Autodesk Inventor part; units mm, degrees
ref_plane "YZ Plane" through (0, 0, 0) normal (1, 0, 0) x (0, 1, 0)
ref_plane "XZ Plane" through (0, 0, 0) normal (0, 1, 0) x (-1, 0, 0)
ref_plane "XY Plane" through (0, 0, 0) normal (0, 0, 1) x (1, 0, 0)
sketch "Sketch44" plane through (0, 0, 0) normal (0, 1, 0) x (-1, 0, 0)
  line L0 (-39.5, 120) -> (39.5, 120)
  line L1 (39.5, 120) -> (39.5, -120)
  line L2 (39.5, -120) -> (-39.5, -120)
  line L3 (-39.5, -120) -> (-39.5, 120)
  line L4 (-39.5, 120) -> (39.5, -120) construction
  line L5 (39.5, 120) -> (-39.5, -120) construction
  point P0 (0, 0)
  dimension "d138" = 79
  dimension "d139" = 240
extrude "Extrusion33" add sketch "Sketch44" along normal blind 3
sketch "Sketch45" plane through (0, 3, 0) normal (0, 1, 0) x (1, 0, 0)
  line L0 (35, -20) -> (-3, -20)
  line L1 (-3, -20) -> (-3, 20)
  line L2 (-3, 20) -> (35, 20)
  line L3 (35, 20) -> (35, -20)
  point P0 (0, 0)
  dimension "d142" = 38
  dimension "d143" = 40
extrude "Extrusion34" add sketch "Sketch45" along normal blind 30
sketch "Sketch46" plane through (0, 33, 0) normal (0, 1, 0) x (1, 0, 0)
  point P0 (0, 0)
sketch "Sketch47" plane through (0, 0, 0) normal (0, -1, 0) x (1, 0, 0)
  circle A0 centre (16, 0) radius 18
  point P0 (0, 0)
  dimension "d146" = 36
extrude "Extrusion35" cut sketch "Sketch47" against normal blind 30 draft -15
sketch "Sketch48" plane through (0, 33, 0) normal (0, 1, 0) x (1, 0, 0)
  point P0 (0, 0)
sketch "Sketch49" plane through (0, 33, 0) normal (0, 1, 0) x (1, 0, 0)
  circle A0 centre (20, 0) radius 0.5
  point P0 (0, 0)
  dimension "d149" = 1
extrude "Extrusion36" cut sketch "Sketch49" against normal through all
sketch "Sketch58" plane through (35, 3, -20) normal (0, 0, -1) x (-1, 0, 0)
  line L0 (7, 20) -> (27, 20)
  line L1 (27, 20) -> (27, 5)
  line L2 (27, 5) -> (7, 5)
  line L3 (7, 5) -> (7, 20)
  point P0 (35, -3)
  dimension "d156" = 20
  dimension "d157" = 15
extrude "Extrusion38" cut sketch "Sketch58" against normal blind 15
sketch "Sketch59" plane through (-3, 3, -20) normal (-1, 0, 0) x (0, 0, 1)
  line L0 (5, 25) -> (8, 25)
  line L1 (8, 25) -> (8, 5)
  line L2 (8, 5) -> (5, 5)
  line L3 (5, 5) -> (5, 25)
  point P0 (20, -3)
  dimension "d160" = 3
  dimension "d161" = 20
extrude "Extrusion39" cut sketch "Sketch59" against normal blind 35
sketch "Sketch60" plane through (0, 3, 0) normal (0, 1, 0) x (1, 0, 0)
  line L0 (-33.965, 38.3247) -> (-28.965, 38.3247)
  line L1 (-28.965, 38.3247) -> (-28.965, 58.3247)
  line L2 (-28.965, 58.3247) -> (-33.965, 58.3247)
  line L3 (-33.965, 58.3247) -> (-33.965, 38.3247)
  point P0 (0, 0)
  dimension "d164" = 5
  dimension "d165" = 20
extrude "Extrusion40" add sketch "Sketch60" along normal blind 20
sketch "Sketch61" plane through (0, 23, 0) normal (0, 1, 0) x (1, 0, 0)
  line L0 (-28.965, 38.3247) -> (-28.965, 58.3247)
  line L1 (-28.965, 38.3247) -> (-48.965, 38.3247)
  line L2 (-48.965, 38.3247) -> (-48.965, 58.3247)
  line L3 (-48.965, 58.3247) -> (-28.965, 58.3247)
  line L4 (-28.965, 58.3247) -> (-28.965, 38.3247)
  point P0 (0, 0)
  dimension "d168" = 20
  dimension "d169" = 20
extrude "Extrusion41" add sketch "Sketch61" against normal blind 5
properties part number "liquid port_v07"
Could you check a few things on this model? Use its own coordinates, in mm. A direction names the side the tool comes from. Give positions to 0.01 mm unless a question says otherwise; leave off trailing zeros. Write each loop counter-clockwise with the first axis right and the second up, starting at its lowest first coordinate (ties: lowest second). Pieces come first, ordered by that corner, then holes. Notation, with made-up numbers: (-36.5, -28) - (-14.5, -28) arc R19 cw to (-14.5, -24) - close; hole circle Ø3 at (-28, 28.5). An arc over 180 degrees is marked (long way). Use CSV: the item, a comma, the result in double quotes. Start each with the question number.
Item 1: If we mould it in two halves opening along Z, with no side actions, what happens to faces 1 (the face through (6, 20, -15)), 2 (the face through (-48.965, 21, -48)), 3 (the face through (16, 18, 20)), 4 (the face through (-32, 17, -58.325))? For each: pulls with the +Z half, pulls with the -Z half, needs draft (parallel to the pull), parting line crosses it, or undercut.
Item 2: For faces 5 (the face through (10, 25, -12)), 6 (the face through (14, 8, -16)), 7 (the face through (28, 17, -9)), which set-ups out of +Z, -Z, +X, -X, +Y, -Y let a thin tool reach every point of the face, with its end or its side?
Item 3: If I drill on line 1 along Z through (x, y) = (20, 32); line 2 along Z through (x, y) = (4, 14.5); line 3 along X through (y, z) = (31.6, 0), over which ranges is the centre line in solid material (lowest first)?
Item 4: I want a section at B-B, the plane z = -79. Please give me the cut outline in (x, y), then the cut area to 3 significant figures.
Item 5: I want a section at A-A, the plane x = 16. Please give me the cut outline in (y, z).
Item 6: I'm going to push flat-ended pins straight in: pin 1 (1.5 mm diameter, centred on y = 2, z = 43.5, fed in from -X); pin 2 (12 mm diameter, centred on x = -30, y = 13, fed in from +Z); pin 3 (16.5 mm diameter, centred on x = -40, z = -45.5, fed in from -Y); pin 4 (1 mm diameter, centred on y = 16, z = 21, fed in from -X). Where does each tip first touch, or does it pass through?
Findings:
1,face 1,"undercut"
1,face 2,"needs draft"
1,face 3,"pulls with the +Z half"
1,face 4,"pulls with the -Z half"
2,face 5,"-X"
2,face 6,"none"
2,face 7,"-Z"
3,line 1,"z = -20 to -0.5, 0.5 to 20"
3,line 2,"z = -20 to -15, -12 to -7.43, 7.43 to 20"
3,line 3,"x = -3 to 19.5, 20.5 to 35"
4,outline,"(-39.5, 0) - (39.5, 0) - (39.5, 3) - (-39.5, 3) - close"
4,area,"237 mm2"
5,outline,"(0, -120) - (3, -120) - (3, -20) - (8, -20) - (8, -15.86) - (0, -18) - close; (0, 18) - (30, 9.96) - (30, -9.96) - (23, -11.84) - (23, -12) - (28, -12) - (28, -15) - (23, -15) - (23, -20) - (33, -20) - (33, 20) - (3, 20) - (3, 120) - (0, 120) - close"
6,pin 1,"stops at x = -39.5"
6,pin 2,"stops at z = -38.32"
6,pin 3,"stops at y = 0"
6,pin 4,"passes through"
